Model file for the job. Use its own axes, mm. Face numbers are marked on the shaded views. A direction names the side the tool comes from. Round coordinates to 2 decimals unless told otherwise and drop trailing zeros. Order: outer loops, then holes, each group sorted by start corner. A loop starts at its lowest first (then second) coordinate and runs counter-clockwise, first axis right, second up. Notation, with made-up numbers: (87.5, 40.25) - (109.5, 40.25) arc R8 cw to (109.5, 45.25) - close; hole circle Ø2 at (39, 88). An arc over 180 degrees is marked (long way). Write item = value, one per line.
```python
from build123d import *

# Parameters (mm, degrees)
F0_R     = 6
F1_DEPTH = 6
F2_R     = 4.5
F3_DEPTH = 30
F4_R     = 2
F6_D     = 6
F6_DEPTH = 15
F6_TIP   = 1.8025818571


with BuildPart() as f1:
    # F0 (on Front) → F1 (new body)
    with BuildSketch(Plane.XZ):
        Circle(F0_R)
    extrude(amount=F1_DEPTH)

    # F2 (on face) → F3 (join)
    with BuildSketch(Plane.XZ.offset(6)):
        Circle(F2_R)
    extrude(amount=F3_DEPTH)

    # F4
    f4_edges = [f1.edges().sort_by_distance(p)[0] for p in [
        (-4.5, -36, 0),
    ]]
    fillet(f4_edges, radius=F4_R)

    # F6
    with Locations(Plane(origin=(0, 0, 0), x_dir=(-1, 0, 0), z_dir=(0, 1, 0))):
        with Locations((0, 0)):
            Hole(F6_D / 2, depth=F6_DEPTH)
            with Locations((0, 0, -(F6_DEPTH + F6_TIP / 2))):  # 118° drill point
                Cone(0, F6_D / 2, F6_TIP, mode=Mode.SUBTRACT)


solid = f1.part
```
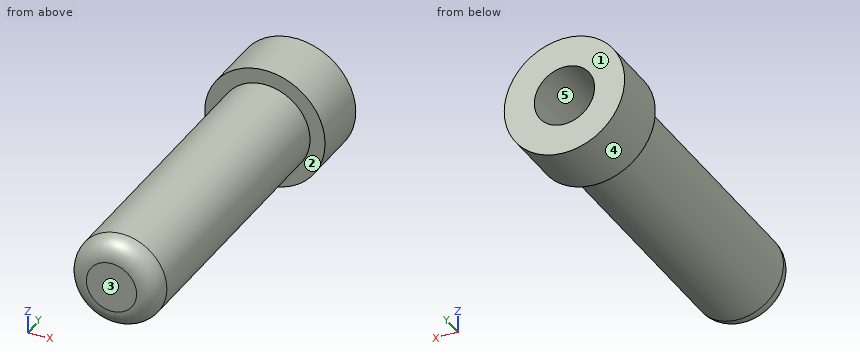
1) 3-axis set-ups, long thin cutter, end or side, ignore diameter. For the marked faces 1 and 2: which of +Z, -Z, +X, -X, +Y, -Y reach the whole face in a straight line?
Conclusion:
face_1 = +Z, -Z, +X, -X, +Y
face_2 = -Y
2) Wall check: line 1 along Z through (x, y) = (0, -11); line 2 along Z through (x, y) = (0, -5); line 3 along Y through (x, z) = (5.25, 1.25). Give the ranges that are in metal, low to high.
Conclusion:
line_1 = -4.5 to -3, 3 to 4.5
line_2 = -6 to -3, 3 to 6
line_3 = -6 to 0
3) Cut at C-C (x = 5.25). Write the cut outline in (y, z).
Conclusion:
outline = (-6, -2.9) - (0, -2.9) - (0, 2.9) - (-6, 2.9) - close
4) Cut at B-B (y = -12.5). Write the cut outline in (x, z).
Conclusion:
outline = circle Ø9 at (0, 0); hole circle Ø6 at (0, 0)
5) Flat gauge pins, fed straight in: pin 1 Ø5 at (x, y) = (0, -20.5) entering from +Z; pin 2 Ø2 at (x, y) = (-3.5, -32) entering from +Z; pin 3 Ø1 at (y, z) = (-19, -4.5) entering from +X. Where does each tip first touch, or does it go through?
Conclusion:
pin_1 = 4.5
pin_2 = 3.74
pin_3 = 2.06
6) Mould opens along X. For the marked faces 3, 4 and 5 say: +X half, -X half, draft (parallel to the pull), parting line (faces both ways), or undercut.
Conclusion:
face_3 = draft
face_4 = parting line
face_5 = undercut
7) Cut at A-A (y = -3). Write the cut outline in (x, z), and give its area (3 significant figures).
Conclusion:
outline = circle Ø12 at (0, 0); hole circle Ø6 at (0, 0)
area = 84.8 mm^2
